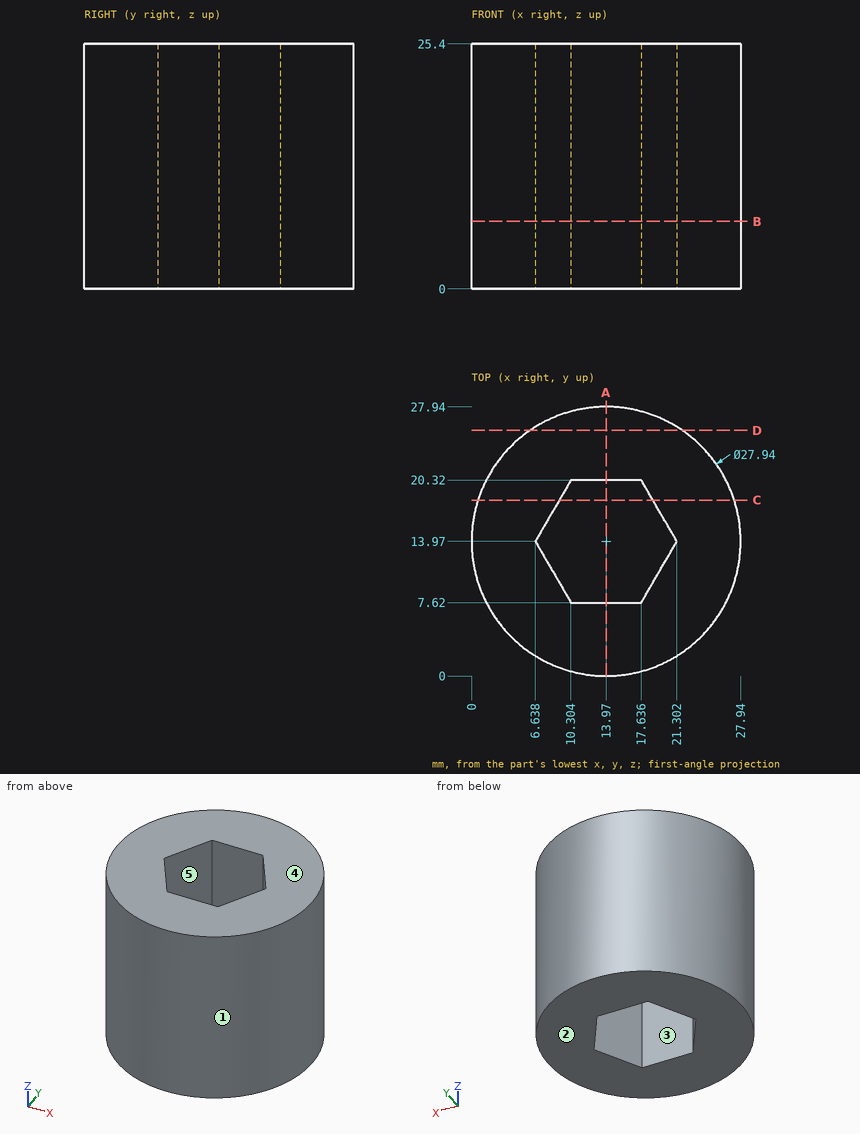
The drawing under review shows one solid part. Ordinate dimensions are in mm from its lowest x, y, z. A direction names the side the tool comes from. Coordinates: 2 decimals unless noted, no trailing zeros. Loops run counter-clockwise (first coordinate to the right, second up) from the corner with the lowest first, then second, coordinate; pieces in that order, holes last.
Item 1: Add section B-B (z = 7). Write out the cut boundary in (x, y).
Completed:
outline: circle Ø27.94 at (13.97, 13.97); hole (6.64, 13.97) - (10.3, 7.62) - (17.64, 7.62) - (21.3, 13.97) - (17.64, 20.32) - (10.3, 20.32) - close
Item 2: Clearance check with flat-ended pins moving along their axes: pin 1 (8 mm diameter, centred on x = 7, z = 7.5, fed in from +Y); pin 2 (8 mm diameter, centred on x = 15.5, z = 10.5, fed in from +Y); pin 3 (6 mm diameter, centred on y = 3, z = 3.5, fed in from +X); pin 4 (4 mm diameter, centred on y = 4.5, z = 16, fed in from -X) (1 decimal). State where each tip first meets the part, or that it passes through.
Completed:
pin 1: stops at y = 27.62
pin 2: stops at y = 27.94
pin 3: stops at x = 25.44
pin 4: stops at x = 2.2
Item 3: Draft analysis for pull direction X (two halves, no side actions). For the marked faces 1, 2 and 3, state which applies: pulls with the +X half, pulls with the -X half, needs draft (parallel to the pull), parting line crosses it, or undercut.
Completed:
face 1: parting line crosses it
face 2: needs draft
face 3: undercut
Item 4: For the marked faces 4 and 5, list the 3-axis set-ups (+Z, -Z, +X, -X, +Y, -Y) from which the entire face can be reached by the end or side of a thin tool; tool diameter is ignored.
Completed:
face 4: +Z, +X, -X, +Y, -Y
face 5: +Z, -Z
Item 5: Add section A-A (x = 13.97). Write out the cut boundary in (y, z), and give its area (3 significant figures).
Completed:
outline: (0, 0) - (7.62, 0) - (7.62, 25.4) - (0, 25.4) - close; (20.32, 0) - (27.94, 0) - (27.94, 25.4) - (20.32, 25.4) - close
area: 387 mm2
Item 6: Add section C-C (y = 18.25). Write out the cut boundary in (x, z), and give its area (3 significant figures).
Completed:
outline: (0.67, 0) - (9.11, 0) - (9.11, 25.4) - (0.67, 25.4) - close; (18.83, 0) - (27.27, 0) - (27.27, 25.4) - (18.83, 25.4) - close
area: 429 mm2
Item 7: Add section D-D (y = 25.5). Write out the cut boundary in (x, z).
Completed:
outline: (6.08, 0) - (21.86, 0) - (21.86, 25.4) - (6.08, 25.4) - close
Item 8: Wall thickness on L1, parallel to Y at x = 14, z = 9.5; L2, parallel to Y at x = 18.25, z = 15.25 (1 decimal); L3, parallel to X at y = 8.25, z = 16 (1 decimal): over which ranges is each line inside the solid? List them lowest first.
Completed:
L1: y = 0 to 7.62, 20.32 to 27.94
L2: y = 0.7 to 8.7, 19.3 to 27.3
L3: x = 1.2 to 9.9, 18 to 26.7
